Work out the finished part from the listing and answer in its coordinate system (mm). A direction names the side the tool comes from. Round coordinates to 2 decimals unless told otherwise and drop trailing zeros. Order: outer loops, then holes, each group sorted by start corner. A loop starts at its lowest first (then second) coordinate and runs counter-clockwise, first axis right, second up. Notation, with made-up numbers: (70, 62) -> (93, 62) arc R20 cw to (93, 68) -> close; hole circle Ø8 at (62, 10.5). An arc over 180 degrees is marked (long way). Use one line per item in the form item = value.
```python
from build123d import *

# Parameters (mm, degrees)
SKETCH1_W           = 77.47
SKETCH1_H           = 52.07
SKETCH1_R           = 1.5875
SKETCH1_H_2         = 52.34
BOSS_EXTRUDE3_DEPTH = 6.35
SKETCH2_W           = 19.05
SKETCH2_H           = 1
CUT_EXTRUDE1_DEPTH  = 193.995155978
SKETCH4_W           = 19.05
SKETCH4_H           = 1
CUT_EXTRUDE2_DEPTH  = 193.995155978
SKETCH5_W           = 257.81
SKETCH5_H           = 1
BOSS_EXTRUDE4_DEPTH = 215.9
SKETCH6_W           = 57.15
SKETCH6_H           = 31.75
CUT_EXTRUDE3_DEPTH  = 193.964841955


with BuildPart() as part:
    # Sketch1 → Boss-Extrude3 (new body)
    with BuildSketch(Plane(origin=(0, 0, 0), x_dir=(1, 0, 0), z_dir=(0, 1, 0))):
        Polygon((148.59, 94.11025641), (129.54, 94.11025641), (129.54, 113.16025641), (-137.02974359, 113.16025641), (-137.02974359, 93.98), (-156.21, 93.98), (-156.21, -88.9), (-137.16, -88.9), (-137.16, -106.95), (-156.21, -106.95), (-156.21, -107.95), (148.59, -107.95), (148.59, -106.95), (129.54, -106.95), (129.54, -88.9), (148.59, -88.9), align=None)
        with Locations((-95.885, -80.915)):
            Rectangle(SKETCH1_W, SKETCH1_H, mode=Mode.SUBTRACT)
        with Locations((-5.715, -80.915)):
            Rectangle(SKETCH1_W, SKETCH1_H, mode=Mode.SUBTRACT)
        with Locations((84.455, -80.915)):
            Rectangle(SKETCH1_W, SKETCH1_H, mode=Mode.SUBTRACT)
        with Locations((84.455, 82.915)):
            Rectangle(SKETCH1_W, SKETCH1_H, mode=Mode.SUBTRACT)
        with Locations((84.455, 28.305)):
            Rectangle(SKETCH1_W, SKETCH1_H, mode=Mode.SUBTRACT)
        with Locations((84.455, -26.305)):
            Rectangle(SKETCH1_W, SKETCH1_H, mode=Mode.SUBTRACT)
        with Locations(Location((139.065, 75.334869264, 0), (0, 0, 270))):
            Circle(SKETCH1_R, mode=Mode.SUBTRACT)
        with Locations(Location((139.065, 80.910552749, 0), (0, 0, 270))):
            Circle(SKETCH1_R, mode=Mode.SUBTRACT)
        with Locations(Location((139.065, 86.618990604, 0), (0, 0, 270))):
            Circle(SKETCH1_R, mode=Mode.SUBTRACT)
        with Locations((-5.715, 82.915)):
            Rectangle(SKETCH1_W, SKETCH1_H, mode=Mode.SUBTRACT)
        with Locations((-95.885, -26.305)):
            Rectangle(SKETCH1_W, SKETCH1_H, mode=Mode.SUBTRACT)
        with Locations((-5.715, -26.17)):
            Rectangle(SKETCH1_W, SKETCH1_H_2, mode=Mode.SUBTRACT)
        with Locations((-95.885, 28.305)):
            Rectangle(SKETCH1_W, SKETCH1_H, mode=Mode.SUBTRACT)
        with Locations((-5.715, 28.305)):
            Rectangle(SKETCH1_W, SKETCH1_H, mode=Mode.SUBTRACT)
        with Locations((-95.885, 82.915)):
            Rectangle(SKETCH1_W, SKETCH1_H, mode=Mode.SUBTRACT)
    extrude(amount=BOSS_EXTRUDE3_DEPTH)

    # Sketch2 → Cut-Extrude1 (cut, through all)
    with BuildSketch(Plane(origin=(0, 6.35, 0), x_dir=(1, 0, 0), z_dir=(0, 1, 0))):
        with Locations((139.065, -107.45)):
            Rectangle(SKETCH2_W, SKETCH2_H)
    extrude(amount=-CUT_EXTRUDE1_DEPTH, mode=Mode.SUBTRACT)

    # Sketch4 → Cut-Extrude2 (cut, through all)
    with BuildSketch(Plane(origin=(0, 6.35, 0), x_dir=(1, 0, 0), z_dir=(0, 1, 0))):
        with Locations((-146.685, -107.45)):
            Rectangle(SKETCH4_W, SKETCH4_H)
    extrude(amount=-CUT_EXTRUDE2_DEPTH, mode=Mode.SUBTRACT)

    # Sketch5 → Boss-Extrude4 (add)
    with BuildSketch(Plane.XY.offset(-108.95)):
        with Locations((-5.715, 0.5)):
            Rectangle(SKETCH5_W, SKETCH5_H)
    extrude(amount=BOSS_EXTRUDE4_DEPTH)

    # Sketch6 → Cut-Extrude3 (cut, through all)
    with BuildSketch(Plane(origin=(0, 1, 0), x_dir=(1, 0, 0), z_dir=(0, 1, 0))):
        with Locations((-95.885, 82.915)):
            Rectangle(SKETCH6_W, SKETCH6_H)
        with Locations((-95.885, 28.305)):
            Rectangle(SKETCH6_W, SKETCH6_H)
        with Locations((-95.885, -26.305)):
            Rectangle(SKETCH6_W, SKETCH6_H)
        with Locations((-95.885, -80.915)):
            Rectangle(SKETCH6_W, SKETCH6_H)
        with Locations((-5.715, 82.915)):
            Rectangle(SKETCH6_W, SKETCH6_H)
        with Locations((84.455, 82.915)):
            Rectangle(SKETCH6_W, SKETCH6_H)
        with Locations((-5.715, 28.305)):
            Rectangle(SKETCH6_W, SKETCH6_H)
        with Locations((-5.715, -26.305)):
            Rectangle(SKETCH6_W, SKETCH6_H)
        with Locations((-5.715, -80.915)):
            Rectangle(SKETCH6_W, SKETCH6_H)
        with Locations((84.455, -80.915)):
            Rectangle(SKETCH6_W, SKETCH6_H)
        with Locations((84.455, -26.305)):
            Rectangle(SKETCH6_W, SKETCH6_H)
        with Locations((84.455, 28.305)):
            Rectangle(SKETCH6_W, SKETCH6_H)
    extrude(amount=-CUT_EXTRUDE3_DEPTH, mode=Mode.SUBTRACT)


solid = part.part
```
Item 1: Flat-ended cylindrical pins translate along their axes: P1, Ø6, axis at x = -40.5, z = -75, coming from the +Y side; P2, Ø2.5, axis at x = 139.06, z = -86.62, coming from the -Y side. Find the tip coordinate at first contact, or state that the pin passes through.
Findings:
P1 = 1
P2 = through
Item 2: The part is cut by section D-D, the plane x = 88.5. Give the number of separate pieces and of enclosed holes in the cut face, and give its area (3 significant figures).
Findings:
separate_pieces = 5
enclosed_holes = 0
area = 163 mm^2
Item 3: The part is cut by section C-C, the plane z = 59. Give the vertices of the cut face in (x, y), and give its area (3 significant figures).
Findings:
outline = (-156.21, 0) -> (148.59, 0) -> (148.59, 6.35) -> (123.19, 6.35) -> (123.19, 1) -> (45.72, 1) -> (45.72, 6.35) -> (33.02, 6.35) -> (33.02, 1) -> (-44.45, 1) -> (-44.45, 6.35) -> (-57.15, 6.35) -> (-57.15, 1) -> (-134.62, 1) -> (-134.62, 6.35) -> (-156.21, 6.35) -> close
area = 692 mm^2
Item 4: Determine the mould class of faces 1 (the flat face through (-2, 3, -113.16)), 2 (the flat face through (84, 1, 9)), 3 (the flat face through (-156.21, 3, -4)) for opening direction X: released by +X, released by -X, zero draft, split by the parting line, or undercut.
Findings:
face_1 = zero draft
face_2 = undercut
face_3 = released by -X
Item 5: The part is cut by section B-B, the plane x = 50. Give the vertices of the cut face in (y, z), and give its area (3 significant figures).
Findings:
outline = (0, -113.16) -> (6.35, -113.16) -> (6.35, -108.95) -> (1, -108.95) -> (1, -56.88) -> (6.35, -56.88) -> (6.35, -54.34) -> (1, -54.34) -> (1, -2.27) -> (6.35, -2.27) -> (6.35, 0.27) -> (1, 0.27) -> (1, 52.34) -> (6.35, 52.34) -> (6.35, 54.88) -> (1, 54.88) -> (1, 106.95) -> (6.35, 106.95) -> (6.35, 107.95) -> (0, 107.95) -> close
area = 290 mm^2
Item 6: Consider line 1 along Z through (x, y) = (8, 4); line 2 along Z through (x, y) = (-127.5, 3); line 3 along X through (y, z) = (4.25, -90). Determine where each line is inside the solid, lowest interval first.
Findings:
line_1 = -113.16 to -108.95, -56.88 to -54.34, -2.27 to 0, 52.34 to 54.88, 106.95 to 107.95
line_2 = -113.16 to -108.95, -56.88 to -54.34, -2.27 to 0.27, 52.34 to 54.88, 106.95 to 107.95
line_3 = -156.21 to -134.62, -57.15 to -44.45, 33.02 to 45.72, 123.19 to 148.59
Item 7: The part is cut by section A-A, the plane z = 14.5. Give the vertices of the cut face in (x, y).
Findings:
outline = (-156.21, 0) -> (-124.46, 0) -> (-124.46, 1) -> (-134.62, 1) -> (-134.62, 6.35) -> (-156.21, 6.35) -> close; (-67.31, 0) -> (-34.29, 0) -> (-34.29, 1) -> (-44.45, 1) -> (-44.45, 6.35) -> (-57.15, 6.35) -> (-57.15, 1) -> (-67.31, 1) -> close; (22.86, 0) -> (55.88, 0) -> (55.88, 1) -> (45.72, 1) -> (45.72, 6.35) -> (33.02, 6.35) -> (33.02, 1) -> (22.86, 1) -> close; (113.03, 0) -> (148.59, 0) -> (148.59, 6.35) -> (123.19, 6.35) -> (123.19, 1) -> (113.03, 1) -> close
Item 8: For faces 4 (the flat face through (129.54, 3, 99)), 5 (the flat face through (-146, 3, -93.98)), 6 (the flat face through (-147, 3, 88.9)), 7 (the flat face through (-96, 1, 63)), 8 (the flat face through (129.54, 3, -104)), determine the directions among +Z, -Z, +X, -X, +Y, -Y from which every point of the face is accessible in a straight line to the end or side of a thin tool.
Findings:
face_4 = +Z, +X, +Y, -Y
face_5 = -Z, -X, +Y, -Y
face_6 = +Z, -X, +Y, -Y
face_7 = +Y
face_8 = -Z, +X, +Y, -Y
